Part model, mm, in its own coordinate system. Face numbers are marked on the shaded views. A direction names the side the tool comes from. Round coordinates to 2 decimals unless told otherwise and drop trailing zeros. Order: outer loops, then holes, each group sorted by start corner. A loop starts at its lowest first (then second) coordinate and runs counter-clockwise, first axis right, second up. Notation, with made-up numbers: (84.5, 41.25) - (138.5, 41.25) arc R18 ccw to (138.5, 76.25) - close; hole circle Ø6 at (78.5, 56). An arc over 180 degrees is marked (long way). Answer as a JSON object with one key per item and string values.
```python
from build123d import *

# Parameters (mm, degrees)
ESQUISSE4_R             = 10
BOSS_EXTRU_3_DEPTH      = 2.5
ESQUISSE5_R             = 0.8
ENL_V_MAT_EXTRU_2_DEPTH = 3
ESQUISSE6_R             = 2.75
ESQUISSE6_R_2           = 1.7
BOSS_EXTRU_4_DEPTH      = 4
ENL_V_START             = -1
ESQUISSE10_R            = 1.7
ENL_V_MAT_EXTRU_3_DEPTH = 1
BOSS_EXTRU_8_START      = -2.5
BOSS_EXTRU_8_DEPTH      = 2.5
ESQUISSE19_R            = 2.5
ENL_V_MAT_EXTRU_4_DEPTH = 3


with BuildPart() as part:
    # Esquisse4 → Boss.-Extru.3 (new body)
    with BuildSketch(Plane.XY):
        Circle(ESQUISSE4_R)
    extrude(amount=BOSS_EXTRU_3_DEPTH)

    # Esquisse5 → Enlèv. mat.-Extru.2 (cut)
    with BuildSketch(Plane.XY.offset(2.5)):
        Circle(ESQUISSE5_R)
    extrude(amount=-ENL_V_MAT_EXTRU_2_DEPTH, mode=Mode.SUBTRACT)

    # Esquisse6 → Boss.-Extru.4 (add)
    with BuildSketch(Plane.XY.offset(2.5)):
        Circle(ESQUISSE6_R)
        Circle(ESQUISSE6_R_2, mode=Mode.SUBTRACT)
    extrude(amount=BOSS_EXTRU_4_DEPTH)

    # Esquisse10 → Enlèv. mat.-Extru.3 (cut)
    with BuildSketch(Plane.XY.offset(2.5).offset(ENL_V_START)):
        Circle(ESQUISSE10_R)
    extrude(amount=ENL_V_MAT_EXTRU_3_DEPTH, mode=Mode.SUBTRACT)

    # Esquisse17 → Boss.-Extru.8 (add)
    with BuildSketch(Plane.XY.offset(2.5).offset(BOSS_EXTRU_8_START)):
        with BuildLine():
            Line((-5, -8.660254038), (-5, -15))
            Line((-5, -15), (5, -15))
            Line((5, -15), (5, -8.660254038))
            ThreePointArc((5, -8.660254038), (0, -10), (-5, -8.660254038))
        make_face()
        with BuildLine():
            Line((5, 15), (5, 8.660254038))
            ThreePointArc((5, 8.660254038), (0, 10), (-5, 8.660254038))
            Line((-5, 8.660254038), (-5, 15))
            Line((-5, 15), (5, 15))
        make_face()
    extrude(amount=BOSS_EXTRU_8_DEPTH)

    # Esquisse19 → Enlèv. mat.-Extru.4 (cut)
    with BuildSketch(Plane.XY.offset(2.5)):
        with Locations((0, -10)):
            Circle(ESQUISSE19_R)
        with Locations((0, 10)):
            Circle(ESQUISSE19_R)
    extrude(amount=-ENL_V_MAT_EXTRU_4_DEPTH, mode=Mode.SUBTRACT)


solid = part.part
```
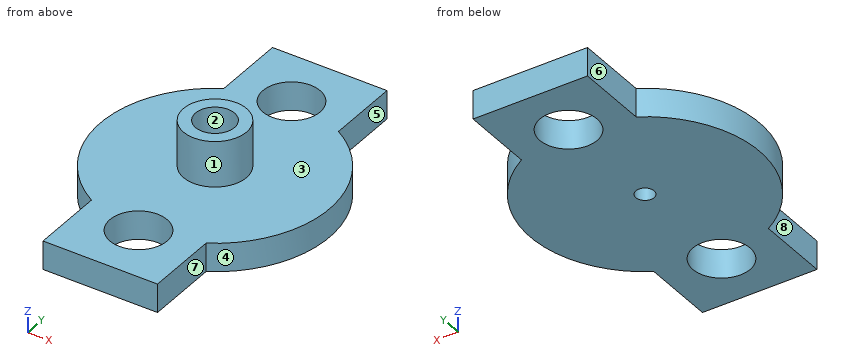
Item 1: Cut at B-B (y = 10). Write the cut outline in (x, z), plus the area to 3 significant figures.
Taken from the geometry:
{"outline": "(-5, 0) - (-2.5, 0) - (-2.5, 2.5) - (-5, 2.5) - close; (2.5, 0) - (5, 0) - (5, 2.5) - (2.5, 2.5) - close", "area": "12.5 mm2"}
Item 2: Cut at C-C (z = 0.5). Write the cut outline in (x, y), plus the area to 3 significant figures.
Taken from the geometry:
{"outline": "(-5, -15) - (5, -15) - (5, -8.66) arc R10 ccw to (5, 8.66) - (5, 15) - (-5, 15) - (-5, 8.66) arc R10 ccw to (-5, -8.66) - close; hole circle Ø5 at (0, -10); hole circle Ø5 at (0, 10); hole circle Ø1.6 at (0, 0)", "area": "382 mm2"}
Item 3: Two-plate mould, pull along X, no slides. Class the marked faces 1, 2, 3 and 4: pulls with the +X half, pulls with the -X half, needs draft (parallel to the pull), parting line crosses it, or undercut.
Taken from the geometry:
{"face 1": "parting line crosses it", "face 2": "undercut", "face 3": "needs draft", "face 4": "pulls with the +X half"}
Item 4: Cut at A-A (x = 0). Write the cut outline in (y, z), plus the area to 3 significant figures.
Taken from the geometry:
{"outline": "(-15, 0) - (-12.5, 0) - (-12.5, 2.5) - (-15, 2.5) - close; (-7.5, 0) - (-0.8, 0) - (-0.8, 1.5) - (-1.7, 1.5) - (-1.7, 6.5) - (-2.75, 6.5) - (-2.75, 2.5) - (-7.5, 2.5) - close; (0.8, 0) - (7.5, 0) - (7.5, 2.5) - (2.75, 2.5) - (2.75, 6.5) - (1.7, 6.5) - (1.7, 1.5) - (0.8, 1.5) - close; (12.5, 0) - (15, 0) - (15, 2.5) - (12.5, 2.5) - close", "area": "52.6 mm2"}
Item 5: Probe L1, parallel to Y at x = 0, z = 0.6; L2, parallel to Y at x = 0, z = 1.85; L3, parallel to Y at x = -1.75, z = 0.75. List the from-to ranges inside material, lowest first. Write a range as from..to.
Taken from the geometry:
{"L1": "-15..-12.5, -7.5..-0.8, 0.8..7.5, 12.5..15", "L2": "-15..-12.5, -7.5..-1.7, 1.7..7.5, 12.5..15", "L3": "-15..-11.79, -8.21..8.21, 11.79..15"}
Item 6: Tool access for the marked faces 5, 6, 7 and 8: list every direction of +Z, -Z, +X, -X, +Y, -Y with a clear straight run to the whole face (end or side of a thin tool).
Taken from the geometry:
{"face 5": "+Z, -Z, +X, +Y", "face 6": "+Z, -Z, -X, +Y", "face 7": "+Z, -Z, +X, -Y", "face 8": "+Z, -Z, -X, -Y"}
Item 7: Drop flat-ended pins along their axis: P1, Ø3, axis at y = 10.5, z = 1, coming from the -X side; P2, Ø0.8, axis at y = 11, z = 1, coming from the +X side; P3, Ø2.5, axis at x = 0, y = 0, coming from the -Z side; P4, Ø1.7, axis at x = 0.5, y = 0, coming from the +Z side. Give the stop position or say it passes through.
Taken from the geometry:
{"P1": "x = -5", "P2": "x = 5", "P3": "z = 0", "P4": "z = 1.5"}
Item 8: Cut at D-D (z = 2). Write the cut outline in (x, y).
Taken from the geometry:
{"outline": "(-5, -15) - (5, -15) - (5, -8.66) arc R10 ccw to (5, 8.66) - (5, 15) - (-5, 15) - (-5, 8.66) arc R10 ccw to (-5, -8.66) - close; hole circle Ø5 at (0, -10); hole circle Ø5 at (0, 10); hole circle Ø3.4 at (0, 0)"}
